```python
from build123d import *

# Parameters (mm, degrees)
F0_W           = 60
F0_H           = 10
F1_DEPTH       = 4
F2_W           = 10
F2_H           = 10
F2_W_2         = 24
F3_DEPTH       = 6
F5_D           = 3
F5_CSINK_D     = 5
F5_CSINK_ANGLE = 90


with BuildPart() as f1:
    # F0 (on Top) → F1 (new body)
    with BuildSketch(Plane.XY):
        Rectangle(F0_W, F0_H)
    extrude(amount=F1_DEPTH)

    # F2 (on face) → F3 (join)
    with BuildSketch(Plane.XY.offset(4)):
        with Locations((-25, 0)):
            Rectangle(F2_W, F2_H)
        Rectangle(F2_W_2, F2_H)
        with Locations((25, 0)):
            Rectangle(F2_W, F2_H)
    extrude(amount=F3_DEPTH)

    # F5 (through all)
    with Locations(Plane(origin=(0, 0, 0), x_dir=(1, 0, 0), z_dir=(0, 0, -1))):
        with Locations((-16, 0), (16, 0)):
            CounterSinkHole(F5_D / 2, F5_CSINK_D / 2, counter_sink_angle=F5_CSINK_ANGLE)


solid = f1.part
```
Build history of the part. All positions in model axes, mm. A direction names the side the tool comes from. Give positions to 0.01 mm unless a question says otherwise; leave off trailing zeros. Loops run counter-clockwise (first coordinate to the right, second up) from the corner with the lowest first, then second, coordinate; pieces in that order, holes last.
1) Probe line 1 along X through (y, z) = (1.25, 6.75); line 2 along Y through (x, z) = (-16, 2.95); line 3 along Z through (x, y) = (12.5, -3.5). List the from-to ranges inside material, lowest first.
Values follow:
line 1: x = -30 to -20, -12 to 12, 20 to 30
line 2: y = -5 to -1.5, 1.5 to 5
line 3: z = 0 to 4
2) Band-saw the part on C-C on z = 8.5. List the corners of the cut face in (x, y), then the cut area to 3 significant figures.
Values follow:
outline: (-30, -5) - (-20, -5) - (-20, 5) - (-30, 5) - close; (-12, -5) - (12, -5) - (12, 5) - (-12, 5) - close; (20, -5) - (30, -5) - (30, 5) - (20, 5) - close
area: 440 mm2
3) 3-axis set-ups, long thin cutter, end or side, ignore diameter. For faces 5 (the face through (12, 0, 7)), 6 (the face through (-14.5, -0.07, 2.52)): which of +Z, -Z, +X, -X, +Y, -Y reach the whole face in a straight line?
Values follow:
face 5: +Z, +Y, -Y
face 6: +Z, -Z
4) Band-saw the part on B-B on x = -16. List the corners of the cut face in (y, z).
Values follow:
outline: (-5, 0) - (-2.5, 0) - (-1.5, 1) - (-1.5, 4) - (-5, 4) - close; (1.5, 1) - (2.5, 0) - (5, 0) - (5, 4) - (1.5, 4) - close
5) Two-plate mould, pull along X, no slides. Class faces 1 (the face through (30, 0, 5)), 2 (the face through (-30, 0, 5)), 3 (the face through (25, 0, 10)), 4 (the face through (-12, 0, 7)): released by +X, released by -X, zero draft, split by the parting line, or undercut.
Values follow:
face 1: released by +X
face 2: released by -X
face 3: zero draft
face 4: undercut
6) Band-saw the part on D-D on y = 3.5. List the corners of the cut face in (x, z), then the cut area to 3 significant figures.
Values follow:
outline: (-30, 0) - (30, 0) - (30, 10) - (20, 10) - (20, 4) - (12, 4) - (12, 10) - (-12, 10) - (-12, 4) - (-20, 4) - (-20, 10) - (-30, 10) - close
area: 504 mm2
7) Drop flat-ended pins along their axis: P1, Ø3, axis at x = 14.5, z = 6, coming from the +Y side; P2, Ø2.5, axis at x = -16, y = -1.5, coming from the +Z side. Give the stop position or say it passes through.
Values follow:
P1: passes through
P2: stops at z = 4
8) Band-saw the part on A-A on y = 0. List the corners of the cut face in (x, z), then the cut area to 3 significant figures.
Values follow:
outline: (-30, 0) - (-18.5, 0) - (-17.5, 1) - (-17.5, 4) - (-20, 4) - (-20, 10) - (-30, 10) - close; (-14.5, 1) - (-13.5, 0) - (13.5, 0) - (14.5, 1) - (14.5, 4) - (12, 4) - (12, 10) - (-12, 10) - (-12, 4) - (-14.5, 4) - close; (17.5, 1) - (18.5, 0) - (30, 0) - (30, 10) - (20, 10) - (20, 4) - (17.5, 4) - close
area: 478 mm2
